from build123d import *

# Parameters (mm, degrees)
BOSS_EXTRUDE1_DEPTH = 7.62
SKETCH2_R           = 3.17999999
CUT_EXTRUDE1_DEPTH  = 45.72
SKETCH3_W           = 17.5
SKETCH3_H           = 38.105
BOSS_EXTRUDE2_DEPTH = 5.99948
FILLET1_R           = 7.5
SKETCH5_R           = 6.75
SKETCH5_R_2         = 7
CUT_EXTRUDE2_DEPTH  = 10
FILLET2_R           = 2


with BuildPart() as part:
    # Sketch1 → Boss-Extrude1 (new body)
    with BuildSketch(Plane.XY):
        Polygon((-95.4, 59.77), (-95.4, 79.77), (163, 79.77), (163, 59.77), (93, 59.77), (93, 6.27), (67.6, 6.27), (67.6, 59.77), (0, 59.77), (0, 6.27), (-25.4, 6.27), (-25.4, 59.77), align=None)
    extrude(amount=BOSS_EXTRUDE1_DEPTH)

    # Sketch2 → Cut-Extrude1 (cut)
    with BuildSketch(Plane(origin=(0, 0, 0), x_dir=(-1, 0, 0), z_dir=(0, 0, -1))):
        with Locations((-80.3, 57.97)):
            Circle(SKETCH2_R)
        with Locations((-80.3, 26.22)):
            Circle(SKETCH2_R)
        with Locations((12.7, 26.22)):
            Circle(SKETCH2_R)
        with Locations((12.7, 57.97)):
            Circle(SKETCH2_R)
    extrude(amount=-CUT_EXTRUDE1_DEPTH, mode=Mode.SUBTRACT)

    # Sketch3 → Boss-Extrude2 (add)
    with BuildSketch(Plane(origin=(0, 79.77, 0), x_dir=(1, 0, 0), z_dir=(0, 1, 0))):
        with Locations((144.8, -26.6725)):
            Rectangle(SKETCH3_W, SKETCH3_H)
        with Locations((-77.2, -26.6725)):
            Rectangle(SKETCH3_W, SKETCH3_H)
        with Locations((-3.2, -26.6725)):
            Rectangle(SKETCH3_W, SKETCH3_H)
        with Locations((70.8, -26.6725)):
            Rectangle(SKETCH3_W, SKETCH3_H)
    extrude(amount=-BOSS_EXTRUDE2_DEPTH)

    # Fillet1
    fillet1_edges = [part.edges().sort_by_distance(p)[0] for p in [
        (-95.4, 59.77, 3.81),
        (-95.4, 79.77, 3.81),
        (163, 79.77, 3.81),
        (163, 59.77, 3.81),
        (93, 59.77, 3.81),
        (93, 6.27, 3.81),
        (67.6, 6.27, 3.81),
        (67.6, 59.77, 3.81),
        (0, 59.77, 3.81),
        (0, 6.27, 3.81),
        (-25.4, 6.27, 3.81),
        (-25.4, 59.77, 3.81),
    ]]
    fillet(fillet1_edges, radius=FILLET1_R)

    # Sketch5 → Cut-Extrude2 (cut)
    with BuildSketch(Plane(origin=(0, 79.77, 0), x_dir=(1, 0, 0), z_dir=(0, 1, 0))):
        with Locations(Location((144.800446227, -34.97274241, 0), (0, 0, 180))):
            Circle(SKETCH5_R)
        with Locations(Location((70.800446272, -34.975332504, 0), (0, 0, 180))):
            Circle(SKETCH5_R_2)
        with Locations(Location((-3.199553683, -34.977922599, 0), (0, 0, 180))):
            Circle(SKETCH5_R_2)
        with Locations(Location((-77.199553637, -34.980512693, 0), (0, 0, 180))):
            Circle(SKETCH5_R_2)
    extrude(amount=-CUT_EXTRUDE2_DEPTH, mode=Mode.SUBTRACT)

    # Fillet2
    fillet2_edges = [part.edges().sort_by_distance(p)[0] for p in [
        (153.55, 76.77026, 7.62),
        (153.55, 76.77026, 45.725),
        (136.05, 76.77026, 45.725),
        (136.05, 76.77026, 7.62),
        (-85.95, 76.77026, 45.725),
        (-85.95, 76.77026, 7.62),
        (-68.45, 76.77026, 7.62),
        (-68.45, 76.77026, 45.725),
        (5.55, 76.77026, 7.62),
        (5.55, 76.77026, 45.725),
        (-11.95, 76.77026, 45.725),
        (-11.95, 76.77026, 7.62),
        (62.05, 76.77026, 7.62),
        (79.55, 76.77026, 7.62),
        (79.55, 76.77026, 45.725),
        (62.05, 76.77026, 45.725),
    ]]
    fillet(fillet2_edges, radius=FILLET2_R)


solid = part.part
Could you check a few things on this model? Use its own coordinates, in mm. A direction names the side the tool comes from. Round coordinates to 2 decimals unless told otherwise and drop trailing zeros. Order: outer loops, then holes, each group sorted by start corner. A loop starts at its lowest first (then second) coordinate and runs counter-clockwise, first axis right, second up.
Q1. Imagine slicing it at D-D, the plane x = 16. List the corners of the cut face in (y, z) for me, then the cut area to 3 significant figures.
Geometry says:
outline: (59.77, 0) - (79.77, 0) - (79.77, 7.62) - (59.77, 7.62) - close
area: 152 mm2
Q2. Which directions (+Z, -Z, +X, -X, +Y, -Y) give clear straight access to the entire face, cutting with the end or side of a thin tool? Please do faces 5 (the face through (5.55, 77, 27)), 6 (the face through (128, 59.77, 4)), 7 (the face through (-60, 59.77, 4)), 8 (the face through (65.345, 57.631, 3.863)).
Geometry says:
face 5: +Z, +Y, -Y
face 6: +Z, -Z, +X, -Y
face 7: +Z, -Z, -X, -Y
face 8: +Z, -Z, -Y
Q3. Please list where these lines run through material, in increasing order: probe 1 along Y at (x, z) = (80.3, 1.75); probe 2 along X at (y, z) = (76.5, 15); probe 3 along Z at (x, y) = (73.5, 68).
Geometry says:
probe 1: y = 6.27 to 23.04, 29.4 to 54.79, 61.15 to 79.77
probe 2: x = -85.95 to -68.45, -11.95 to 5.55, 62.05 to 79.55, 136.05 to 153.55
probe 3: z = 0 to 7.62
Q4. I'm going to push flat-ended pins straight in: P1, Ø12.5, axis at x = -3.2, z = 34.98, coming from the -Y side; P2, Ø17, axis at x = 0, z = 29, coming from the -Y side; P3, Ø5, axis at y = 77.5, z = 26, coming from the +X side; P4, Ø3, axis at y = 75.5, z = 27.5, coming from the -X side. Where does each tip first touch, or does it pass through?
Geometry says:
P1: passes through
P2: stops at y = 73.77
P3: stops at x = 153.55
P4: stops at x = -85.95
Q5. Imagine slicing it at B-B, the plane z = 14.5. List the corners of the cut face in (x, y) for me.
Geometry says:
outline: (-85.95, 73.77) - (-68.45, 73.77) - (-68.45, 79.77) - (-85.95, 79.77) - close; (-11.95, 73.77) - (5.55, 73.77) - (5.55, 79.77) - (-11.95, 79.77) - close; (62.05, 73.77) - (79.55, 73.77) - (79.55, 79.77) - (62.05, 79.77) - close; (136.05, 73.77) - (153.55, 73.77) - (153.55, 79.77) - (136.05, 79.77) - close
Q6. Imagine slicing it at C-C, the plane y = 11. List the corners of the cut face in (x, z) for me.
Geometry says:
outline: (-24.87, 0) - (-0.53, 0) - (-0.53, 7.62) - (-24.87, 7.62) - close; (68.13, 0) - (92.47, 0) - (92.47, 7.62) - (68.13, 7.62) - close
Q7. Imagine slicing it at A-A, the plane y = 26.22. List the corners of the cut face in (x, z) for me.
Geometry says:
outline: (-25.4, 0) - (-15.88, 0) - (-15.88, 7.62) - (-25.4, 7.62) - close; (-9.52, 0) - (0, 0) - (0, 7.62) - (-9.52, 7.62) - close; (67.6, 0) - (77.12, 0) - (77.12, 7.62) - (67.6, 7.62) - close; (83.48, 0) - (93, 0) - (93, 7.62) - (83.48, 7.62) - close
Q8. Thinking about a two-plate mould opening in X: for faces 1 (the face through (71, 73.771, 22)), 2 (the face through (-14.17, 55.15, 3.76)), 3 (the face through (93, 33, 4)), 4 (the face through (2.139, 57.515, 3.863)), which applies, released by +X, released by -X, zero draft, split by the parting line, or undercut?
Geometry says:
face 1: zero draft
face 2: undercut
face 3: released by +X
face 4: undercut
